Input: dimensioned drawing with shaded views. Units: mm. Origin: part minimum x, y, z. Coordinates: 2 decimals unless noted, no trailing zeros. Loops run counter-clockwise (first coordinate to the right, second up) from the corner with the lowest first, then second, coordinate; pieces in that order, holes last. Notation, with made-up numbers: (-11.75, 47.5) - (9.25, 47.5) arc R25 ccw to (9.25, 70.5) - close; hole circle Ø5 at (40.25, 40). An arc over 180 degrees is marked (long way). Put each result on its own line as item: value. Start each with the question number.
1) Section B-B on z = 8.25. Output: boundary loops of the cut face in (x, y), and give its area (3 significant figures).
2) Draft query along X for the marked faces 1, 2, 3 and 4. Return one class per face: +X half, -X half, draft (parallel to the pull), parting line (faces both ways), or undercut.
3) Section D-D on y = 42. Output: boundary loops of the cut face in (x, z).
4) Section C-C on x = 21. Output: boundary loops of the cut face in (y, z), and give its area (3 significant figures).
5) Material intervals for line 1 along Y through (x, z) = (21, 5); line 2 along Y through (x, z) = (37, 2.75); line 3 along Y through (x, z) = (20, 7.5), sorted ascending. Write a range as from..to.
6) Contact query for a flat-ended pin moving along its axis: pin 1 Ø4 at (x, y) = (37, 7.5) entering from +Z (3 decimals). Output: stop coordinate, or through.
7) Section A-A on x = 38. Output: boundary loops of the cut face in (y, z).
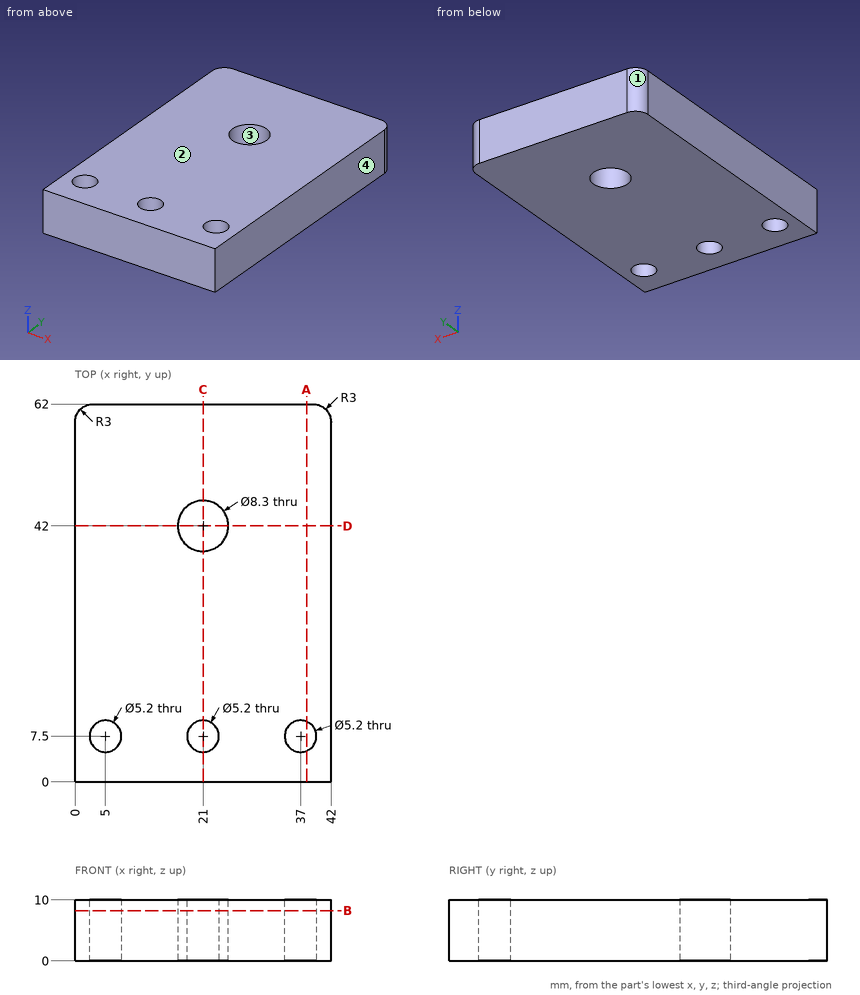
Answer block:
1. outline: (0, 0) - (42, 0) - (42, 59) arc R3 ccw to (39, 62) - (3, 62) arc R3 ccw to (0, 59) - close; hole circle Ø5.2 at (5, 7.5); hole circle Ø8.3 at (21, 42); hole circle Ø5.2 at (21, 7.5); hole circle Ø5.2 at (37, 7.5)
1. area: 2,480 mm²
2. face 1: -X half
2. face 2: draft
2. face 3: undercut
2. face 4: +X half
3. outline: (0, 0) - (16.85, 0) - (16.85, 10) - (0, 10) - close; (25.15, 0) - (42, 0) - (42, 10) - (25.15, 10) - close
4. outline: (0, 0) - (4.9, 0) - (4.9, 10) - (0, 10) - close; (10.1, 0) - (37.85, 0) - (37.85, 10) - (10.1, 10) - close; (46.15, 0) - (62, 0) - (62, 10) - (46.15, 10) - close
4. area: 485 mm²
5. line 1: y = 0..4.9, 10.1..37.85, 46.15..62
5. line 2: y = 0..4.9, 10.1..62
5. line 3: y = 0..5.1, 9.9..37.97, 46.03..62
6. pin 1: passes through
7. outline: (0, 0) - (5.1, 0) - (5.1, 10) - (0, 10) - close; (9.9, 0) - (62, 0) - (62, 10) - (9.9, 10) - close
